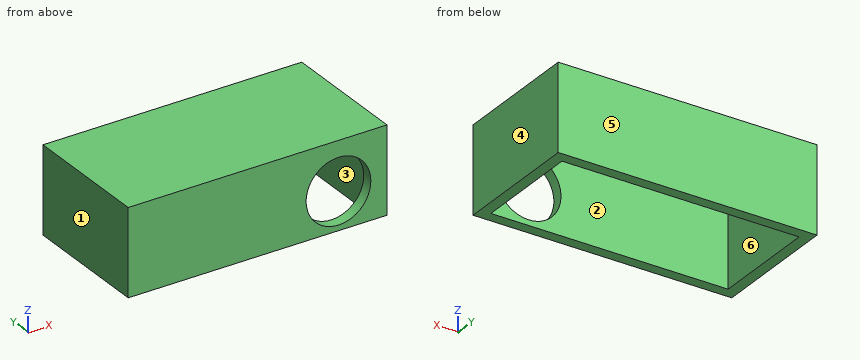
```python
from build123d import *

# Parameters (mm, degrees)
F0_W     = 304.8
F0_H     = 101.6
F1_DEPTH = 76.2
F2_W     = 279.4
F2_H     = 127
F3_DEPTH = 88.9
F4_R     = 38.1
F5_DEPTH = 12.7


with BuildPart() as f1:
    # F0 (on Front) → F1 (new body, symmetric)
    with BuildSketch(Plane.XZ):
        Rectangle(F0_W, F0_H)
    extrude(amount=F1_DEPTH, both=True)

    # F2 (on face) → F3 (cut)
    with BuildSketch(Plane(origin=(0, 0, -50.8), x_dir=(1, 0, 0), z_dir=(0, 0, -1))):
        Rectangle(F2_W, F2_H)
    extrude(amount=-F3_DEPTH, mode=Mode.SUBTRACT)

    # F4 (on face) → F5 (cut)
    with BuildSketch(Plane.XZ.offset(76.2)):
        with Locations((95.25, -6.35)):
            Circle(F4_R)
    extrude(amount=-F5_DEPTH, mode=Mode.SUBTRACT)


solid = f1.part
```
Source: CAD feature listing. Evaluate the final solid. Frame: model axes, mm. Face numbers are marked on the shaded views. A direction names the side the tool comes from. Give positions to 0.01 mm unless a question says otherwise; leave off trailing zeros. Order: outer loops, then holes, each group sorted by start corner. A loop starts at its lowest first (then second) coordinate and runs counter-clockwise, first axis right, second up.
(1) Section query B-B (y = -46). Return the cut outline in (x, z), plus the area to 3 significant figures.
(2) Section query C-C (x = 28.5). Return the cut outline in (y, z), plus the area to 3 significant figures.
(3) Section query A-A (x = 95.25). Return the cut outline in (y, z), plus the area to 3 significant figures.
(4) Access query for the marked faces 5 and 6. Directions: +Z, -Z, +X, -X, +Y, -Y. A direction counts if a zero-diameter tool reaches every point of the face in a straight line with its end or side. Return the directions, or none.
(5) Material intervals for line 1 along X through (y, z) = (27, -17); line 2 along Z through (x, y) = (95.25, -66.5); line 3 along X through (y, z) = (-72, -6), sorted ascending.
(6) Pull-direction query (X, two-part tool) for the marked faces 1, 2, 3 and 4; classes: +X half, -X half, draft (parallel to the pull), parting line (faces both ways), or undercut.
(7) Contact query for a flat-ended pin moving along its axis: P1, Ø10, axis at x = -100.5, y = 38.5, coming from the -Z side. Output: stop coordinate, or through.
(8) Section query D-D (z = -6.35). Return the cut outline in (x, y).
Outcome:
1. outline: (-152.4, -50.8) - (-139.7, -50.8) - (-139.7, 38.1) - (139.7, 38.1) - (139.7, -50.8) - (152.4, -50.8) - (152.4, 50.8) - (-152.4, 50.8) - close
1. area: 6,130 mm2
2. outline: (-76.2, -50.8) - (-63.5, -50.8) - (-63.5, 38.1) - (63.5, 38.1) - (63.5, -50.8) - (76.2, -50.8) - (76.2, 50.8) - (-76.2, 50.8) - close
2. area: 4,190 mm2
3. outline: (-76.2, -50.8) - (-63.5, -50.8) - (-63.5, -44.45) - (-76.2, -44.45) - close; (-76.2, 31.75) - (-63.5, 31.75) - (-63.5, 38.1) - (63.5, 38.1) - (63.5, -50.8) - (76.2, -50.8) - (76.2, 50.8) - (-76.2, 50.8) - close
3. area: 3,230 mm2
4. face 5: +Z, -Z, +X, -X, +Y
4. face 6: -Z
5. line 1: x = -152.4 to -139.7, 139.7 to 152.4
5. line 2: z = -50.8 to -44.45, 31.75 to 50.8
5. line 3: x = -152.4 to 57.15, 133.35 to 152.4
6. face 1: -X half
6. face 2: undercut
6. face 3: undercut
6. face 4: +X half
7. P1: stops at z = 38.1
8. outline: (-152.4, -76.2) - (57.15, -76.2) - (57.15, -63.5) - (-139.7, -63.5) - (-139.7, 63.5) - (139.7, 63.5) - (139.7, -63.5) - (133.35, -63.5) - (133.35, -76.2) - (152.4, -76.2) - (152.4, 76.2) - (-152.4, 76.2) - close
